Could you check a few things on this model? Use its own coordinates, in mm. A direction names the side the tool comes from. Coordinates: 2 decimals unless noted, no trailing zeros. Loops run counter-clockwise (first coordinate to the right, second up) from the corner with the lowest first, then second, coordinate; pieces in that order, holes last. Notation, with made-up numbers: (63, -11) - (104, -11) arc R21 ccw to (104, 19) - close; hole circle Ø3 at (84.25, 75). An arc over 180 degrees is marked (long way). One line per question, with ' | ' between items. Start each with the question number.
1. I want a section at A-A, the plane y = 7.75. Write out the boundary of the cut face in (x, z), then the cut area to 3 significant figures.
2. Which directions (+Z, -Z, +X, -X, +Y, -Y) give clear straight access to the entire face, cutting with the end or side of a thin tool? Please do faces 1 (the flat face through (-2.155, 2.465, -3.663)), 2 (the flat face through (10, 9.8, -0.4)), 3 (the flat face through (0.14, 10.818, -13.131)), 4 (the flat face through (-16.6, 3, 14.9)).
3. I want a section at C-C, the plane y = 1.25. Write out the boundary of the cut face in (x, z), then the cut area to 3 significant figures.
4. I'm going to push flat-ended pins straight in: P1, Ø3, axis at x = 18.5, z = 16.5, coming from the +Y side; P2, Ø1.5, axis at x = -5, z = 1.5, coming from the -Y side; P3, Ø4, axis at x = 20, z = -15, coming from the -Y side; P4, Ø10, axis at x = -21.5, z = 19, coming from the +Y side. Where does each tip first touch, or does it pass through?
5. I want a section at B-B, the plane x = 17.5. Write out the boundary of the cut face in (y, z).
6. Please list where these lines run through material, in increasing order: L1, parallel to X at y = 7, z = 15; L2, parallel to X at y = 1.15, z = -15; L3, parallel to Z at x = 24, y = 5.5. Write a range as [from, to].
from build123d import *

# Parameters (mm, degrees)
SKETCH1_W           = 56
SKETCH1_H           = 60
SKETCH1_R           = 3.25
BOSS_EXTRUDE1_DEPTH = 3
SKETCH2_W           = 56
SKETCH2_H           = 60
SKETCH2_R           = 5.25
BOSS_EXTRUDE2_DEPTH = 6
FILLET1_R           = 6
BOSS_EXTRUDE3_DEPTH = 10
SKETCH4_R           = 2.75
CUT_EXTRUDE2_DEPTH  = 43.700231647
SKETCH5_R           = 3.5
CUT_EXTRUDE3_DEPTH  = 43.011903097
CUT_EXTRUDE4_DEPTH  = 5


with BuildPart() as part:
    # Sketch1 → Boss-Extrude1 (new body)
    with BuildSketch(Plane(origin=(0, 0, 0), x_dir=(1, 0, 0), z_dir=(0, 1, 0))):
        Rectangle(SKETCH1_W, SKETCH1_H)
        with Locations(Location((-20, 15, 0), (0, 0, 270))):
            Circle(SKETCH1_R, mode=Mode.SUBTRACT)
        with Locations(Location((-20, -15, 0), (0, 0, 270))):
            Circle(SKETCH1_R, mode=Mode.SUBTRACT)
        with Locations(Location((20, -15, 0), (0, 0, 270))):
            Circle(SKETCH1_R, mode=Mode.SUBTRACT)
        with Locations(Location((20, 15, 0), (0, 0, 270))):
            Circle(SKETCH1_R, mode=Mode.SUBTRACT)
    extrude(amount=BOSS_EXTRUDE1_DEPTH)

    # Sketch2 → Boss-Extrude2 (add)
    with BuildSketch(Plane(origin=(0, 3, 0), x_dir=(1, 0, 0), z_dir=(0, 1, 0))):
        Rectangle(SKETCH2_W, SKETCH2_H)
        with Locations(Location((-20, 15, 0), (0, 0, 270))):
            Circle(SKETCH2_R, mode=Mode.SUBTRACT)
        with Locations(Location((-20, -15, 0), (0, 0, 270))):
            Circle(SKETCH2_R, mode=Mode.SUBTRACT)
        with Locations(Location((20, -15, 0), (0, 0, 270))):
            Circle(SKETCH2_R, mode=Mode.SUBTRACT)
        with Locations(Location((20, 15, 0), (0, 0, 270))):
            Circle(SKETCH2_R, mode=Mode.SUBTRACT)
    extrude(amount=BOSS_EXTRUDE2_DEPTH)

    # Fillet1
    fillet1_edges = [part.edges().sort_by_distance(p)[0] for p in [
        (28, 4.5, 30),
        (-28, 4.5, 30),
        (-28, 4.5, -30),
        (28, 4.5, -30),
    ]]
    fillet(fillet1_edges, radius=FILLET1_R)

    # Sketch3 → Boss-Extrude3 (add, symmetric)
    with BuildSketch(Plane(origin=(0, 0, 0), x_dir=(0, 0, -1), z_dir=(1, 0, 0))):
        with BuildLine():
            Line((-26, 9), (-26, 10))
            Line((-26, 10), (-24.75, 10))
            Line((-24.75, 10), (-23.976576947, 11.65861109))
            ThreePointArc((-23.976576947, 11.65861109), (-23.75, 11.802956525), (-23.523423053, 11.65861109))
            Line((-23.523423053, 11.65861109), (-22.75, 10))
            ThreePointArc((-22.75, 10), (-22.5, 9.840732435), (-22.25, 10))
            Line((-22.25, 10), (-21.476576947, 11.65861109))
            ThreePointArc((-21.476576947, 11.65861109), (-21.25, 11.802956525), (-21.023423053, 11.65861109))
            Line((-21.023423053, 11.65861109), (-20.25, 10))
            ThreePointArc((-20.25, 10), (-20, 9.840732435), (-19.75, 10))
            Line((-19.75, 10), (-18.976576947, 11.65861109))
            ThreePointArc((-18.976576947, 11.65861109), (-18.75, 11.802956525), (-18.523423053, 11.65861109))
            Line((-18.523423053, 11.65861109), (-17.75, 10))
            ThreePointArc((-17.75, 10), (-17.5, 9.840732435), (-17.25, 10))
            Line((-17.25, 10), (-16.476576947, 11.65861109))
            ThreePointArc((-16.476576947, 11.65861109), (-16.25, 11.802956525), (-16.023423053, 11.65861109))
            Line((-16.023423053, 11.65861109), (-15.25, 10))
            ThreePointArc((-15.25, 10), (-15, 9.840732435), (-14.75, 10))
            Line((-14.75, 10), (-13.976576947, 11.65861109))
            ThreePointArc((-13.976576947, 11.65861109), (-13.75, 11.802956525), (-13.523423053, 11.65861109))
            Line((-13.523423053, 11.65861109), (-12.75, 10))
            ThreePointArc((-12.75, 10), (-12.5, 9.840732435), (-12.25, 10))
            Line((-12.25, 10), (-11.476576947, 11.65861109))
            ThreePointArc((-11.476576947, 11.65861109), (-11.25, 11.802956525), (-11.023423053, 11.65861109))
            Line((-11.023423053, 11.65861109), (-10.25, 10))
            ThreePointArc((-10.25, 10), (-10, 9.840732435), (-9.75, 10))
            Line((-9.75, 10), (-8.976576947, 11.65861109))
            ThreePointArc((-8.976576947, 11.65861109), (-8.75, 11.802956525), (-8.523423053, 11.65861109))
            Line((-8.523423053, 11.65861109), (-7.75, 10))
            ThreePointArc((-7.75, 10), (-7.5, 9.840732435), (-7.25, 10))
            Line((-7.25, 10), (-6.476576947, 11.65861109))
            ThreePointArc((-6.476576947, 11.65861109), (-6.25, 11.802956525), (-6.023423053, 11.65861109))
            Line((-6.023423053, 11.65861109), (-5.25, 10))
            ThreePointArc((-5.25, 10), (-5, 9.840732435), (-4.75, 10))
            Line((-4.75, 10), (-3.976576947, 11.65861109))
            ThreePointArc((-3.976576947, 11.65861109), (-3.75, 11.802956525), (-3.523423053, 11.65861109))
            Line((-3.523423053, 11.65861109), (-2.75, 10))
            ThreePointArc((-2.75, 10), (-2.5, 9.840732435), (-2.25, 10))
            Line((-2.25, 10), (-1.476576947, 11.65861109))
            ThreePointArc((-1.476576947, 11.65861109), (-1.25, 11.802956525), (-1.023423053, 11.65861109))
            Line((-1.023423053, 11.65861109), (-0.25, 10))
            ThreePointArc((-0.25, 10), (0, 9.840732435), (0.25, 10))
            Line((0.25, 10), (1.023423053, 11.65861109))
            ThreePointArc((1.023423053, 11.65861109), (1.25, 11.802956525), (1.476576947, 11.65861109))
            Line((1.476576947, 11.65861109), (2.25, 10))
            ThreePointArc((2.25, 10), (2.5, 9.840732435), (2.75, 10))
            Line((2.75, 10), (3.523423053, 11.65861109))
            ThreePointArc((3.523423053, 11.65861109), (3.75, 11.802956525), (3.976576947, 11.65861109))
            Line((3.976576947, 11.65861109), (4.75, 10))
            ThreePointArc((4.75, 10), (5, 9.840732435), (5.25, 10))
            Line((5.25, 10), (6.023423053, 11.65861109))
            ThreePointArc((6.023423053, 11.65861109), (6.25, 11.802956525), (6.476576947, 11.65861109))
            Line((6.476576947, 11.65861109), (7.25, 10))
            ThreePointArc((7.25, 10), (7.5, 9.840732435), (7.75, 10))
            Line((7.75, 10), (8.523423053, 11.65861109))
            ThreePointArc((8.523423053, 11.65861109), (8.75, 11.802956525), (8.976576947, 11.65861109))
            Line((8.976576947, 11.65861109), (9.75, 10))
            ThreePointArc((9.75, 10), (10, 9.840732435), (10.25, 10))
            Line((10.25, 10), (11.023423053, 11.65861109))
            ThreePointArc((11.023423053, 11.65861109), (11.25, 11.802956525), (11.476576947, 11.65861109))
            Line((11.476576947, 11.65861109), (12.25, 10))
            ThreePointArc((12.25, 10), (12.5, 9.840732435), (12.75, 10))
            Line((12.75, 10), (13.523423053, 11.65861109))
            ThreePointArc((13.523423053, 11.65861109), (13.75, 11.802956525), (13.976576947, 11.65861109))
            Line((13.976576947, 11.65861109), (14.75, 10))
            ThreePointArc((14.75, 10), (15, 9.840732435), (15.25, 10))
            Line((15.25, 10), (16.023423053, 11.65861109))
            ThreePointArc((16.023423053, 11.65861109), (16.25, 11.802956525), (16.476576947, 11.65861109))
            Line((16.476576947, 11.65861109), (17.25, 10))
            ThreePointArc((17.25, 10), (17.5, 9.840732435), (17.75, 10))
            Line((17.75, 10), (18.523423053, 11.65861109))
            ThreePointArc((18.523423053, 11.65861109), (18.75, 11.802956525), (18.976576947, 11.65861109))
            Line((18.976576947, 11.65861109), (19.75, 10))
            ThreePointArc((19.75, 10), (20, 9.840732435), (20.25, 10))
            Line((20.25, 10), (21.023423053, 11.65861109))
            ThreePointArc((21.023423053, 11.65861109), (21.25, 11.802956525), (21.476576947, 11.65861109))
            Line((21.476576947, 11.65861109), (22.25, 10))
            ThreePointArc((22.25, 10), (22.5, 9.840732435), (22.75, 10))
            Line((22.75, 10), (23.523423053, 11.65861109))
            ThreePointArc((23.523423053, 11.65861109), (23.75, 11.802956525), (23.976576947, 11.65861109))
            Line((23.976576947, 11.65861109), (24.75, 10))
            Line((24.75, 10), (26, 10))
            Line((26, 10), (26, 9))
            Line((26, 9), (-26, 9))
        make_face()
    extrude(amount=BOSS_EXTRUDE3_DEPTH, both=True)

    # Sketch4 → Cut-Extrude2 (cut, through all)
    with BuildSketch(Plane(origin=(0, 0, 0), x_dir=(1, 0, 0), z_dir=(0, 1, 0))):
        with Locations(Location((0, 0, 0), (0, 0, 90.000000079))):
            Circle(SKETCH4_R)
    extrude(amount=CUT_EXTRUDE2_DEPTH, mode=Mode.SUBTRACT)

    # Sketch5 → Cut-Extrude3 (cut, through all)
    with BuildSketch(Plane(origin=(0, 9, 0), x_dir=(1, 0, 0), z_dir=(0, 1, 0))):
        with Locations(Location((0, 0, 0), (0, 0, 128.213210702))):
            Circle(SKETCH5_R)
    extrude(amount=CUT_EXTRUDE3_DEPTH, mode=Mode.SUBTRACT)

    # Sketch6 → Cut-Extrude4 (cut)
    with BuildSketch(Plane.XZ):
        Polygon((4.25, -2.453738644), (4.25, 2.453738644), (0, 4.907477288), (-4.25, 2.453738644), (-4.25, -2.453738644), (0, -4.907477288), align=None)
    extrude(amount=-CUT_EXTRUDE4_DEPTH, mode=Mode.SUBTRACT)


solid = part.part
Results are:
1) outline: (-28, -24) arc R6 ccw to (-22, -30) - (22, -30) arc R6 ccw to (28, -24) - (28, 24) arc R6 ccw to (22, 30) - (-22, 30) arc R6 ccw to (-28, 24) - close; hole circle Ø10.5 at (-20, -15); hole circle Ø10.5 at (-20, 15); hole circle Ø5.5 at (0, 0); hole circle Ø10.5 at (20, -15); hole circle Ø10.5 at (20, 15) | area: 2,960 mm2
2) face 1: -Y | face 2: +Z, -Z, +X, +Y | face 3: +X, -X, +Y | face 4: +Y
3) outline: (-28, -24) arc R6 ccw to (-22, -30) - (22, -30) arc R6 ccw to (28, -24) - (28, 24) arc R6 ccw to (22, 30) - (-22, 30) arc R6 ccw to (-28, 24) - close; hole circle Ø6.5 at (-20, -15); hole circle Ø6.5 at (-20, 15); hole (-4.25, -2.45) - (0, -4.91) - (4.25, -2.45) - (4.25, 2.45) - (0, 4.91) - (-4.25, 2.45) - close; hole circle Ø6.5 at (20, -15); hole circle Ø6.5 at (20, 15) | area: 3,130 mm2
4) P1: stops at y = 3 | P2: stops at y = 0 | P3: passes through | P4: stops at y = 9
5) outline: (0, -30) - (9, -30) - (9, -19.62) - (3, -19.62) - (3, -17.08) - (0, -17.08) - close; (0, -12.92) - (3, -12.92) - (3, -10.38) - (9, -10.38) - (9, 10.38) - (3, 10.38) - (3, 12.92) - (0, 12.92) - close; (0, 17.08) - (3, 17.08) - (3, 19.62) - (9, 19.62) - (9, 30) - (0, 30) - close
6) L1: x = [-28, -25.25], [-14.75, 14.75], [25.25, 28] | L2: x = [-28, -23.25], [-16.75, 16.75], [23.25, 28] | L3: z = [-29.66, -18.4], [-11.6, 11.6], [18.4, 29.66]
